Could you check a few things on this model? Use its own coordinates, in mm. Face numbers are marked on the shaded views. A direction names the side the tool comes from. Give positions to 0.01 mm unless a question says otherwise; leave off trailing zeros. Loops run counter-clockwise (first coordinate to the right, second up) from the corner with the lowest first, then second, coordinate; pieces in that order, holes last. Notation, with made-up numbers: (-22, -19.5) - (16, -19.5) arc R33 ccw to (16, 17.5) - close; hole circle Ø2 at (54.5, 54.25). An arc over 180 degrees is marked (long way). Answer in a Markdown table with one row per item. Add a question column.
```python
from build123d import *

# Parameters (mm, degrees)
EXTRUDE_1_DEPTH     = 2.5
FILLET_1_R          = 2.5
SKETCH_4_R          = 1.501202813
CUT_EXTRUDE_2_DEPTH = 5
SKETCH_5_R          = 1.499820195
CUT_EXTRUDE_3_DEPTH = 5
EXTRUDE_START       = -5
SKETCH_6_R          = 1.500762706
EXTRUDE_2_DEPTH     = 5
FILLET_2_R          = 5


with BuildPart() as part:
    # 草图1 → 凸台-拉伸1 (new, symmetric)
    with BuildSketch(Plane.XY):
        with BuildLine():
            Line((0, 9.998744027), (4.99606171, 9.998744027))
            Line((4.99606171, 9.998744027), (4.99606171, 13.997916296))
            Line((4.99606171, 13.997916296), (0, 13.997916296))
            ThreePointArc((0, 13.997916296), (-9.898021536, 9.898021536), (-13.997916296, 0))
            Line((-13.997916296, 0), (-13.997916296, -4.997048222))
            Line((-13.997916296, -4.997048222), (-10.001933758, -4.997048222))
            Line((-10.001933758, -4.997048222), (-10.001933758, 0))
            ThreePointArc((-10.001933758, 0), (-7.072241637, 7.071307535), (0, 9.998744027))
        make_face()
    extrude(amount=EXTRUDE_1_DEPTH, both=True)

    # 圆角1
    fillet_1_edges = [part.edges().sort_by_distance(p)[0] for p in [
        (-11.999925027, -4.997048222, -2.5),
        (-11.999925027, -4.997048222, 2.5),
        (4.99606171, 11.998330162, -2.5),
        (4.99606171, 11.998330162, 2.5),
    ]]
    fillet(fillet_1_edges, radius=FILLET_1_R - 0.0001)  # a hair under: the kernel refuses the full size

    # 草图4 → 切除-拉伸2 (cut)
    with BuildSketch(Plane(origin=(0, 13.997916296, 0), x_dir=(1, 0, 0), z_dir=(0, 1, 0))):
        with Locations(Location((2.49606171, 0, 0), (0, 0, 180))):
            Circle(SKETCH_4_R)
    extrude(amount=-CUT_EXTRUDE_2_DEPTH, mode=Mode.SUBTRACT)

    # 草图5 → 切除-拉伸3 (cut)
    with BuildSketch(Plane.ZY.offset(13.997916296)):
        with Locations((0, -2.497048222)):
            Circle(SKETCH_5_R)
    extrude(amount=-CUT_EXTRUDE_3_DEPTH, mode=Mode.SUBTRACT)

    # 草图6 → 凸台-拉伸2 (add)
    with BuildSketch(Plane(origin=(0, 0, -2.5), x_dir=(-1, 0, 0), z_dir=(0, 0, -1)).offset(EXTRUDE_START)):
        with BuildLine():
            Line((9.898430706, 9.897612349), (16.10800673, 16.291078939))
            ThreePointArc((16.10800673, 16.291078939), (21.958821842, 20.907611506), (20.772449798, 13.549831148))
            Line((20.772449798, 13.549831148), (13.997916296, 0))
            ThreePointArc((13.997916296, 0), (12.932499084, 5.356503344), (9.898430706, 9.897612349))
        make_face()
        with Locations((19.932570399, 17.459789485)):
            Circle(SKETCH_6_R, mode=Mode.SUBTRACT)
    extrude(amount=EXTRUDE_2_DEPTH)

    # 圆角2
    fillet_2_edges = [part.edges().sort_by_distance(p)[0] for p in [
        (-13.997916296, 0, 0),
        (-9.898430706, 9.897612349, 0),
        (-16.10800673, 16.291078939, 0),
        (-20.772449798, 13.549831148, 0),
    ]]
    fillet(fillet_2_edges, radius=FILLET_2_R)


solid = part.part
```
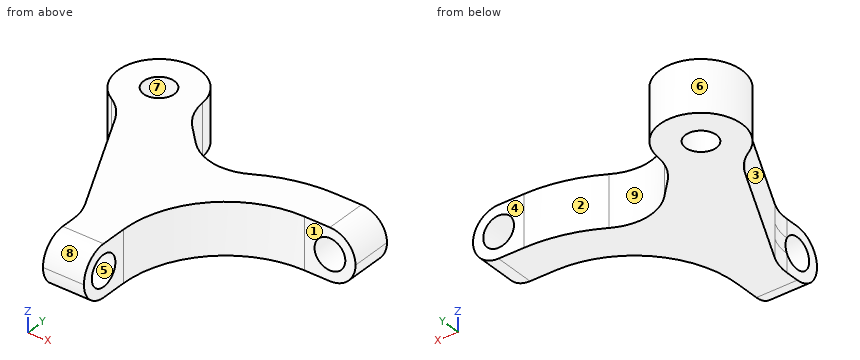
(1) On a 3-axis mill with a long thin cutter (end or side, diameter ignored), from which of +Z, -Z, +X, -X, +Y, -Y can I reach the whole of each face in a straight line? I mean the marked faces 1, 2, 3, 4 and 5. Say none if no direction works.
(2) Please list where these lines run through material, in increasing order: line 1 (Z direction, x = -11, y = -2.5); line 2 (X direction, y = -3, z = -2.05); line 3 (Y direction, x = -19.25, z = 1.15).
(3) I want a section at A-A on x = -9.5. Please give me the cut outline in (y, z).
(4) I want a section at B-B on y = 4.25. Please give me the cut outline in (x, z).
(5) We'd pull the mould along X, two halves only. Please class the marked faces 6, 7, 8 and 9: pulls with the +X half, pulls with the -X half, needs draft (parallel to the pull), parting line crosses it, or undercut.
(6) For pin 1 Ø2.5 at (x, z) = (1.5, 0) entering from -Y; pin 2 Ø1.5 at (y, z) = (-3, 1) entering from +X, each with a flat end and sliding along its axis, tell me the tip position at first contact or that it passes through.
Reported:
| question | item | result |
|---|---|---|
| 1 | face 1 | +Z, -Z, +X, -Y |
| 1 | face 2 | +Z, -Z, +Y |
| 1 | face 3 | +Z, -Z, -X, -Y |
| 1 | face 4 | +Z, -Z, +X, +Y |
| 1 | face 5 | +X, -X |
| 2 | line 1 | -2.5 to -1.5, 1.5 to 2.5 |
| 2 | line 2 | -14 to -10 |
| 2 | line 3 | 10.5 to 16.12, 18.8 to 21.4 |
| 3 | outline | (3.13, -2.5) - (11.53, -2.5) - (11.53, 2.5) - (3.13, 2.5) - close |
| 4 | outline | (-16.12, -2.5) - (-9.05, -2.5) - (-9.05, 2.5) - (-16.12, 2.5) - close |
| 5 | face 6 | parting line crosses it |
| 5 | face 7 | undercut |
| 5 | face 8 | needs draft |
| 5 | face 9 | undercut |
| 6 | pin 1 | y = 10 |
| 6 | pin 2 | x = -10 |
